Source: CAD feature listing. Evaluate the final solid. Frame: model axes, mm. A direction names the side the tool comes from. Coordinates: 2 decimals unless noted, no trailing zeros. Write each loop counter-clockwise with the first axis right and the second up, starting at its lowest first coordinate (ties: lowest second). Pieces come first, ordered by that corner, then holes. Notation, with made-up numbers: M 49,15 L 81,15 A20 ccw 81,33 Z; hole C 56.5,8 d7. An arc over 180 degrees is marked long. Answer as CSV lines item,"result". Start each with the question number.
1. Section C-C on z = -21.5. Return the cut outline in (x, y).
2. Line query: probe 1 along Z at (x, y) = (2, 24); probe 2 along Z at (x, y) = (23.5, 0.5); probe 3 along Y at (x, z) = (28, -10.5). Output: solid intervals per line, ascending. Write a range as [from, to].
3. Contact query for flat-ended pins moving along their axis: pin 1 Ø9.5 at (x, y) = (28, 20.5) entering from +Z; pin 2 Ø2 at (x, y) = (14, -4) entering from +Z. Output: stop coordinate, or through.
4. Section B-B on y = 21.5. Return the cut outline in (x, z), plus the area to 3 significant figures.
5. Reachability of faces 1 (the face through (20, 2, -35.533)), 2 (the face through (23.238, 20.417, -20.97)), 3 (the face through (15, 19, -17.533)) from +Z, -Z, +X, -X, +Y, -Y: full face, straight path, thin tool, end or side. Return the list, or none.
6. Section D-D on x = 26. Return the cut outline in (y, z).
7. Section A-A on x = 4.5. Return the cut outline in (y, z).
```python
from build123d import *

# Parameters (mm, degrees)
F1_DEPTH = 40
F2_W     = 12
F2_H     = 18
F3_DEPTH = 6
F7_DEPTH = 25.4
F8_DEPTH = 13.462
F9_DEPTH = 31.496


with BuildPart() as f1:
    # F0 (on Right) → F1 (new body)
    with BuildSketch(Plane.YZ):
        Polygon((-23.4989325106, -35.5329651147), (14.5010674894, -35.5329651147), (14.5010674894, -17.5329651147), (-11.4989325106, -2.5329651147), (-23.4989325106, -2.5329651147), align=None)
    extrude(amount=F1_DEPTH)

    # F2 (on face) → F3 (join)
    with BuildSketch(Plane(origin=(0, 0, 0), x_dir=(0, -1, 0), z_dir=(-1, 0, 0))):
        with Locations((-20.5010674894, -26.5329651147)):
            Rectangle(F2_W, F2_H)
    extrude(amount=-F3_DEPTH)

    # F5 (on face) → F7 (join)
    with BuildSketch(Plane(origin=(0, 26.5010674894, 0), x_dir=(-1, 0, 0), z_dir=(0, 1, 0))):
        Polygon((-40, -35.5329651147), (-6, -35.5329651147), (-6, -17.5329651147), align=None)
    extrude(amount=-F7_DEPTH)

    # F4 (on face) → F8 (join)
    with BuildSketch(Plane.XY.offset(-17.5329651147)):
        Polygon((6, 26.5010674894), (6, 14.5010674894), (40, 14.5010674894), align=None)
    extrude(amount=-F8_DEPTH)

    # F6 (on face) → F9 (join)
    with BuildSketch(Plane.YZ.offset(40)):
        Polygon((14.5010674894, -17.5329651147), (14.5010674894, -35.5329651147), (26.5010674894, -35.5329651147), align=None)
    extrude(amount=-F9_DEPTH)


solid = f1.part
```
Values:
1,outline,"M 0,-23.5 L 40,-23.5 L 40,17.15 L 32.51,17.15 L 13.49,23.86 L 13.49,26.5 L 0,26.5 Z"
2,probe 1,"[-35.53, -17.53]"
2,probe 2,"[-35.53, -9.46]"
2,probe 3,"[-23.5, 2.31]"
3,pin 1,"z = -17.53"
3,pin 2,"z = -6.28"
4,outline,"M 0,-35.53 L 40,-35.53 L 40,-28.03 L 25.83,-28.03 L 20.17,-25.03 L 20.17,-17.53 L 0,-17.53 Z"
4,area,"520 mm²"
5,face 1,"-Z, +X, -X, +Y, -Y"
5,face 2,"+Z, +X, +Y"
5,face 3,"+Z, +X, -X, +Y"
6,outline,"M -23.5,-35.53 L 26.5,-35.53 L 26.5,-28.12 L 21.56,-28.12 L 19.44,-24.94 L 19.44,-17.53 L 14.5,-17.53 L -11.5,-2.53 L -23.5,-2.53 Z"
7,outline,"M -23.5,-35.53 L 26.5,-35.53 L 26.5,-17.53 L 14.5,-17.53 L -11.5,-2.53 L -23.5,-2.53 Z"
